```python
from build123d import *

# Parameters (mm, degrees)
F1_DEPTH = 26
F2_R     = 2.5
F3_DEPTH = 1
F5_DEPTH = 9.1093520504


with BuildPart() as f1:
    # F0 (on Right) → F1 (new body)
    with BuildSketch(Plane.YZ):
        Polygon((0, 0), (0, 11), (-3.4348489251, 11), (-6, 3.9523053441), (-20, 9.894952771), (-20, 0), align=None)
    extrude(amount=F1_DEPTH)

    # F2 (on face) → F3 (cut)
    with BuildSketch(Plane(origin=(0, -6.5683797818, 2.3906947279), x_dir=(1, 0, 0), z_dir=(0, -0.9396926208, 0.3420201433))):
        with Locations((22.5, 6.161831307)):
            Circle(F2_R)
    extrude(amount=-F3_DEPTH, mode=Mode.SUBTRACT)

    # F4 (on face) → F5 (cut, through all)
    with BuildSketch(Plane(origin=(0, 0.5055003799, 1.190884266), x_dir=(1, 0, 0), z_dir=(0, 0.3907311285, 0.9205048535))):
        with BuildLine():
            Line((26, -7.067317848), (25, -10.067317848))
            ThreePointArc((25, -10.067317848), (13, -17.067317848), (1, -10.067317848))
            Line((1, -10.067317848), (0, -7.067317848))
            Line((0, -7.067317848), (0, -22.2763631316))
            Line((0, -22.2763631316), (26, -22.2763631316))
            Line((26, -22.2763631316), (26, -7.067317848))
        make_face()
    extrude(amount=-F5_DEPTH, mode=Mode.SUBTRACT)


solid = f1.part
```
CAD build for the part. Positions are in the model's coordinates, mm. A direction names the side the tool comes from. Coordinates: 2 decimals unless noted, no trailing zeros. Order: outer loops, then holes, each group sorted by start corner. A loop starts at its lowest first (then second) coordinate and runs counter-clockwise, first axis right, second up. Notation, with made-up numbers: (65, 71) - (89, 71) arc R19 cw to (89, 93) - close; hole circle Ø2 at (1.25, 67). An arc over 180 degrees is marked (long way). Use a Markdown table: item, result. Add a question column.
(1) Saw through at B-B (y = -6.5). Give the cut face in (x, z).
(2) Pull direction X, two halves, no side cores. Call faces 3 (the face through (26, -3, 4)), 4 (the face through (20, -4, 8)), 5 (the face through (13.204, -16.551, 4.684)), 6 (the face through (22.5, -3.5, 7.9)): +X half, -X half, draft (parallel to the pull), parting line (faces both ways), or undercut.
(3) Flat gauge pins, fed straight in: pin 1 (4 mm diameter, centred on x = 9, z = 7.5, fed in from -Y); pin 2 (10 mm diameter, centred on x = 14, y = -13.5, fed in from -Z); pin 3 (3 mm diameter, centred on y = -16.5, z = 4, fed in from -X). Where does each tip first touch, or does it go through?
(4) Saw through at A-A (x = 14.25). Give the cut face in (y, z), then the cut area to 3 significant figures.
(5) Drill centre lines: line 1 along Y through (x, z) = (12.25, 7.5); line 2 along Y through (x, z) = (2, 10); line 3 along X through (y, z) = (-13, 4.25). Where is each one in solid material? Low to high. Write a range as [from, to].
(6) Which spindle directions (+Z, -Z, +X, -X, +Y, -Y) get a long thin tool onto all of the face, cutting with end or side? Do faces 1 (the face through (12.818, -4.699, 7.525)), 2 (the face through (25.51, -8.43, 2)). Say none if no direction does.
Solved:
| question | item | result |
|---|---|---|
| 1 | outline | (0, 0) - (26, 0) - (26, 2.77) - (25.82, 4.16) - (0.18, 4.16) - (0, 2.77) - close |
| 2 | face 3 | +X half |
| 2 | face 4 | undercut |
| 2 | face 5 | parting line |
| 2 | face 6 | undercut |
| 3 | pin 1 | stops at y = -15.73 |
| 3 | pin 2 | stops at z = 0 |
| 3 | pin 3 | stops at x = 6.16 |
| 4 | outline | (-18.48, 0) - (0, 0) - (0, 11) - (-3.43, 11) - (-6, 3.95) - (-15.15, 7.84) - close |
| 4 | area | 124 mm² |
| 5 | line 1 | y = [-15.34, -14.36], [-4.71, 0] |
| 5 | line 2 | y = [-3.8, 0] |
| 5 | line 3 | x = [3.89, 22.11] |
| 6 | face 1 | +Z, +X, -X |
| 6 | face 2 | +Z, +X, -Y |
